```python
from build123d import *

# Parameters (mm, degrees)
SKETCH_1_R          = 80
EXTRUDE_1_DEPTH     = 2.5
SKETCH_2_W          = 100.60548239
SKETCH_2_H          = 145.735598162
CUT_EXTRUDE_1_DEPTH = 114.164702978
SKETCH_3_R          = 2
CUT_EXTRUDE_2_DEPTH = 101.031245119
SKETCH_4_R          = 2
SKETCH_4_W          = 15.232799914
SKETCH_4_H          = 10.431121385
SKETCH_4_W_2        = 11.994997095
SKETCH_4_H_2        = 36
CUT_EXTRUDE_3_DEPTH = 101.031245119
EXTRUDE_2_DEPTH     = 4
SKETCH_6_W          = 32
SKETCH_6_H          = 14.029347869
EXTRUDE_3_DEPTH     = 2
SKETCH_7_R          = 2.217818609
CUT_EXTRUDE_4_DEPTH = 3
SKETCH_8_W          = 28
SKETCH_8_H          = 15.27806524
CUT_EXTRUDE_5_DEPTH = 3


with BuildPart() as part:
    # 草圖1 → 填料-伸長1 (new body)
    with BuildSketch(Plane.XY):
        Circle(SKETCH_1_R)
    extrude(amount=EXTRUDE_1_DEPTH)

    # 草圖2 → 除料-伸長1 (cut, through all)
    with BuildSketch(Plane.XY.offset(2.5)):
        with Locations((110.302741195, -4.321910255)):
            Rectangle(SKETCH_2_W, SKETCH_2_H)
        with Locations((-110.302741195, -4.321910255)):
            Rectangle(SKETCH_2_W, SKETCH_2_H)
    extrude(amount=-CUT_EXTRUDE_1_DEPTH, mode=Mode.SUBTRACT)

    # 草圖3 → 除料-伸長2 (cut, through all)
    with BuildSketch(Plane.XY.offset(2.5)):
        with Locations((50.5, 53)):
            Circle(SKETCH_3_R)
        with Locations(Location((-51.940924548, 53, 0), (0, 0, 180))):
            Circle(SKETCH_3_R)
        with Locations(Location((50.5, -53, 0), (0, 0, 180))):
            Circle(SKETCH_3_R)
        with Locations((-51.940924548, -53)):
            Circle(SKETCH_3_R)
    extrude(amount=-CUT_EXTRUDE_2_DEPTH, mode=Mode.SUBTRACT)

    # 草圖4 → 除料-伸長3 (cut, through all)
    with BuildSketch(Plane.XY.offset(2.5)):
        with Locations((56.024944143, 42.913378777)):
            Circle(SKETCH_4_R)
        with Locations((50, 42.913378777)):
            Circle(SKETCH_4_R)
        with Locations((44, 42.913378777)):
            Circle(SKETCH_4_R)
        with Locations((55.994997095, 24.413403016)):
            Circle(SKETCH_4_R)
        with Locations((50, 24.413403016)):
            Circle(SKETCH_4_R)
        with Locations((44, 24.413403016)):
            Circle(SKETCH_4_R)
        with Locations((-30.354317412, 9.25)):
            Circle(SKETCH_4_R)
        with Locations(Location((30.145682588, 9.25, 0), (0, 0, 180))):
            Circle(SKETCH_4_R)
        with Locations((30.145682588, -9.25)):
            Circle(SKETCH_4_R)
        with Locations(Location((-30.354317412, -9.25, 0), (0, 0, 180))):
            Circle(SKETCH_4_R)
        with Locations((30.145682588, -25.25)):
            Circle(SKETCH_4_R)
        with Locations((30.145682588, -31.25)):
            Circle(SKETCH_4_R)
        with Locations((30.145682588, -37.25)):
            Circle(SKETCH_4_R)
        with Locations(Location((1.145682588, 37.25, 0), (0, 0, 180))):
            Circle(SKETCH_4_R)
        with Locations(Location((1.145682588, 31.25, 0), (0, 0, 180))):
            Circle(SKETCH_4_R)
        with Locations(Location((1.145682588, 25.25, 0), (0, 0, 180))):
            Circle(SKETCH_4_R)
        with Locations((1.145682588, -25.25)):
            Circle(SKETCH_4_R)
        with Locations((1.145682588, -31.25)):
            Circle(SKETCH_4_R)
        with Locations((1.145682588, -37.25)):
            Circle(SKETCH_4_R)
        with Locations(Location((30.145682588, 37.25, 0), (0, 0, 180))):
            Circle(SKETCH_4_R)
        with Locations(Location((30.145682588, 31.25, 0), (0, 0, 180))):
            Circle(SKETCH_4_R)
        with Locations(Location((30.145682588, 25.25, 0), (0, 0, 180))):
            Circle(SKETCH_4_R)
        with Locations(Location((44, -42.913378777, 0), (0, 0, 180))):
            Circle(SKETCH_4_R)
        with Locations(Location((50, -42.913378777, 0), (0, 0, 180))):
            Circle(SKETCH_4_R)
        with Locations(Location((56.024944143, -42.913378777, 0), (0, 0, 180))):
            Circle(SKETCH_4_R)
        with Locations(Location((55.994997095, -24.413403016, 0), (0, 0, 180))):
            Circle(SKETCH_4_R)
        with Locations(Location((50, -24.413403016, 0), (0, 0, 180))):
            Circle(SKETCH_4_R)
        with Locations(Location((44, -24.413403016, 0), (0, 0, 180))):
            Circle(SKETCH_4_R)
        with Locations(Location((-44.208634825, 24.413403016, 0), (0, 0, 180))):
            Circle(SKETCH_4_R)
        with Locations(Location((-50.208634825, 24.413403016, 0), (0, 0, 180))):
            Circle(SKETCH_4_R)
        with Locations(Location((-56.20363192, 24.413403016, 0), (0, 0, 180))):
            Circle(SKETCH_4_R)
        with Locations(Location((-44.208634825, 42.913378777, 0), (0, 0, 180))):
            Circle(SKETCH_4_R)
        with Locations(Location((-50.208634825, 42.913378777, 0), (0, 0, 180))):
            Circle(SKETCH_4_R)
        with Locations(Location((-56.233578968, 42.913378777, 0), (0, 0, 180))):
            Circle(SKETCH_4_R)
        with Locations((-44.208634825, -24.413403016)):
            Circle(SKETCH_4_R)
        with Locations((-50.208634825, -24.413403016)):
            Circle(SKETCH_4_R)
        with Locations((-56.20363192, -24.413403016)):
            Circle(SKETCH_4_R)
        with Locations((-56.233578968, -42.913378777)):
            Circle(SKETCH_4_R)
        with Locations((-50.208634825, -42.913378777)):
            Circle(SKETCH_4_R)
        with Locations((-44.208634825, -42.913378777)):
            Circle(SKETCH_4_R)
        with Locations((50.378597138, 33.525369531)):
            Rectangle(SKETCH_4_W, SKETCH_4_H)
        Polygon((-55.327205732, 17.335052239), (-54.897151983, -18.662378972), (-42.903010794, -18.519087487), (-43.333064544, 17.478343724), align=None)
        with Locations((49.997498548, 0)):
            Rectangle(SKETCH_4_W_2, SKETCH_4_H_2)
        with Locations((50.378597138, -33.525369531)):
            Rectangle(SKETCH_4_W, SKETCH_4_H)
        with Locations((-50.587231963, 33.525369531)):
            Rectangle(SKETCH_4_W, SKETCH_4_H)
        with Locations((-50.587231963, -33.525369531)):
            Rectangle(SKETCH_4_W, SKETCH_4_H)
    extrude(amount=-CUT_EXTRUDE_3_DEPTH, mode=Mode.SUBTRACT)

    # 草圖5 → 填料-伸長2 (add)
    with BuildSketch(Plane.XY.offset(2.5)):
        Polygon((14, 78.029347869), (16, 78.029347869), (16, 66), (16, 64), (-16, 64), (-16, 66), (-16, 78.029347869), (-14, 78.029347869), (-14, 76), (-14, 66), (14, 66), (14, 76), align=None)
    extrude(amount=EXTRUDE_2_DEPTH)

    # 草圖6 → 填料-伸長3 (add)
    with BuildSketch(Plane.XY.offset(6.5)):
        with Locations((0, 71.014673934)):
            Rectangle(SKETCH_6_W, SKETCH_6_H)
    extrude(amount=EXTRUDE_3_DEPTH)

    # 草圖7 → 除料-伸長4 (cut)
    with BuildSketch(Plane.XY.offset(8.5)):
        with Locations((-0.104317412, 72)):
            Circle(SKETCH_7_R)
        with Locations((5.895682588, 72)):
            Circle(SKETCH_7_R)
        with Locations((-6.104317412, 72)):
            Circle(SKETCH_7_R)
    extrude(amount=-CUT_EXTRUDE_4_DEPTH, mode=Mode.SUBTRACT)

    # 草圖8 → 除料-伸長5 (cut)
    with BuildSketch(Plane(origin=(0, 0, 0), x_dir=(-1, 0, 0), z_dir=(0, 0, -1))):
        with Locations((0, 74.312512391)):
            Rectangle(SKETCH_8_W, SKETCH_8_H)
    extrude(amount=-CUT_EXTRUDE_5_DEPTH, mode=Mode.SUBTRACT)


solid = part.part
```
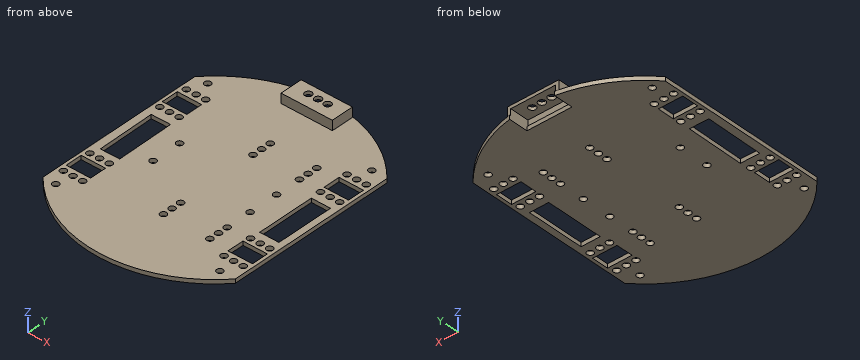
Here's how the part is built. I have some questions about the finished solid (model axes, mm). Give positions to 0.01 mm unless a question says otherwise; leave off trailing zeros. Loops run counter-clockwise (first coordinate to the right, second up) from the corner with the lowest first, then second, coordinate; pieces in that order, holes last. Notation, with made-up numbers: M -28.75,63 L -3.75,63 A27 cw -3.75,90 Z; hole C -21,89 d3. An arc over 180 degrees is marked long. Put each result on its own line as item: value. Start each with the question number.
(1) I want a section at C-C on x = -25.5. Please give me the cut outline in (y, z), then the cut area to 3 significant figures.
(2) Will these pins go through, and if not, where does the flat tip stop? pin 1 Ø4.5 at (x, y) = (-56.2, 24.41) entering from +Z; pin 2 Ø2.5 at (x, y) = (-50.21, 24.41) entering from +Z; pin 3 Ø4.5 at (x, z) = (3, 5) entering from +Y; pin 4 Ø3 at (x, z) = (48.5, 1) entering from -Y.
(3) I want a section at D-D on y = -60. Please give me the cut outline in (x, z).
(4) I want a section at B-B on y = 0.5. Please give me the cut outline in (x, z) (3 decimals), then the cut area to 3 significant figures.
(5) I need wall thicknesses on line 1 along Y through (x, z) = (15, 3.5); line 2 along Z through (x, y) = (-22, 12); line 3 along X through (y, z) = (54.5, 1.75). Which ranges of each line are inside material? Lowest first, please. Write a range as [from, to].
(6) I want a section at A-A on y = -31.25. Please give me the cut outline in (x, z) (3 decimals), then the cut area to 3 significant figures.
Answer block:
1. outline: M -75.83,0 L 75.83,0 L 75.83,2.5 L -75.83,2.5 Z
1. area: 379 mm^2
2. pin 1: z = 2.5
2. pin 2: through
2. pin 3: y = 78.03
2. pin 4: y = -64.74
3. outline: M -52.92,0 L 52.92,0 L 52.92,2.5 L -52.92,2.5 Z
4. outline: M -60,0 L -55.126,0 L -55.126,2.5 L -60,2.5 Z; M -43.13,0 L 44,0 L 44,2.5 L -43.13,2.5 Z; M 55.995,0 L 60,0 L 60,2.5 L 55.995,2.5 Z
4. area: 240 mm^2
5. line 1: [64, 78.03]
5. line 2: [0, 2.5]
5. line 3: [-58.56, -53.26], [-50.62, 49.18], [51.82, 58.56]
6. outline: M -60,0 L -58.204,0 L -58.204,2.5 L -60,2.5 Z; M -42.971,0 L -0.854,0 L -0.854,2.5 L -42.971,2.5 Z; M 3.146,0 L 28.146,0 L 28.146,2.5 L 3.146,2.5 Z; M 32.146,0 L 42.762,0 L 42.762,2.5 L 32.146,2.5 Z; M 57.995,0 L 60,0 L 60,2.5 L 57.995,2.5 Z
6. area: 204 mm^2
